from build123d import *

# Parameters (mm, degrees)
SKETCH1_W           = 2
SKETCH1_H           = 12
SKETCH1_W_2         = 19.5
SKETCH1_H_2         = 27
BOSS_EXTRUDE1_DEPTH = 4
SKETCH2_W           = 19.5
SKETCH2_H           = 5
SKETCH2_R           = 6
BOSS_EXTRUDE2_DEPTH = 16
BOSS_EXTRUDE3_START = 4
SKETCH3_R           = 10
BOSS_EXTRUDE3_DEPTH = 8
CHAMFER1_SIZE       = 1


with BuildPart() as part:
    # Sketch1 → Boss-Extrude1 (new body)
    with BuildSketch(Plane(origin=(0, 0, 0), x_dir=(1, 0, 0), z_dir=(0, 1, 0))):
        with Locations((-10.75, 0)):
            Rectangle(SKETCH1_W, SKETCH1_H)
        Rectangle(SKETCH1_W_2, SKETCH1_H_2)
        with Locations((10.75, 0)):
            Rectangle(SKETCH1_W, SKETCH1_H)
    extrude(amount=BOSS_EXTRUDE1_DEPTH)

    # Sketch2 → Boss-Extrude2 (add)
    with BuildSketch(Plane(origin=(0, 4, 0), x_dir=(1, 0, 0), z_dir=(0, 1, 0))):
        with BuildLine():
            Line((-6.373397172, 3.5), (-4.873397172, 3.5))
            ThreePointArc((-4.873397172, 3.5), (0, 6), (4.873397172, 3.5))
            Line((4.873397172, 3.5), (6.373397172, 3.5))
            Line((6.373397172, 3.5), (9.75, 8.5))
            Line((9.75, 8.5), (-9.75, 8.5))
            Line((-9.75, 8.5), (-6.373397172, 3.5))
        make_face()
        with Locations((0, 11)):
            Rectangle(SKETCH2_W, SKETCH2_H)
        Circle(SKETCH2_R)
        with BuildLine():
            Line((-6.373397172, -3.5), (-9.75, -8.5))
            Line((-9.75, -8.5), (9.75, -8.5))
            Line((9.75, -8.5), (6.373397172, -3.5))
            Line((6.373397172, -3.5), (4.873397172, -3.5))
            ThreePointArc((4.873397172, -3.5), (0, -6), (-4.873397172, -3.5))
            Line((-4.873397172, -3.5), (-6.373397172, -3.5))
        make_face()
        with Locations((0, -11)):
            Rectangle(SKETCH2_W, SKETCH2_H)
    extrude(amount=BOSS_EXTRUDE2_DEPTH)

    # Sketch3 → Boss-Extrude3 (add)
    with BuildSketch(Plane(origin=(0, 4, 0), x_dir=(1, 0, 0), z_dir=(0, 1, 0)).offset(BOSS_EXTRUDE3_START)):
        Circle(SKETCH3_R)
    extrude(amount=BOSS_EXTRUDE3_DEPTH)

    # Chamfer1
    chamfer1_edges = [part.edges().sort_by_distance(p)[0] for p in [
        (-9.75, 10, -13.5),
        (9.75, 10, -13.5),
        (9.75, 10, 13.5),
        (-9.75, 10, 13.5),
    ]]
    chamfer(chamfer1_edges, length=CHAMFER1_SIZE)


solid = part.part
For this review, take the finished solid that the model builds, in its own axes (mm). A direction names the side the tool comes from. Round coordinates to 2 decimals unless told otherwise and drop trailing zeros. Loops run counter-clockwise (first coordinate to the right, second up) from the corner with the lowest first, then second, coordinate; pieces in that order, holes last. Notation, with made-up numbers: (80, 87) - (137, 87) arc R9 ccw to (137, 103) - close; hole circle Ø6 at (-36, 75). An arc over 180 degrees is marked (long way). Use one line per item in the form item = value.
Item 1: Consider section C-C on z = -1.75. Write out the cut boundary in (x, y).
Answers:
outline = (-11.75, 0) - (11.75, 0) - (11.75, 4) - (5.74, 4) - (5.74, 8) - (9.85, 8) - (9.85, 16) - (5.74, 16) - (5.74, 20) - (-5.74, 20) - (-5.74, 16) - (-9.85, 16) - (-9.85, 8) - (-5.74, 8) - (-5.74, 4) - (-11.75, 4) - close
Item 2: Consider section D-D on y = 11.25. Write out the cut boundary in (x, z).
Answers:
outline = (-9.75, -12.5) - (-8.75, -13.5) - (8.75, -13.5) - (9.75, -12.5) - (9.75, -8.5) - (8.03, -5.96) arc R10 ccw to (8.03, 5.96) - (9.75, 8.5) - (9.75, 12.5) - (8.75, 13.5) - (-8.75, 13.5) - (-9.75, 12.5) - (-9.75, 8.5) - (-8.03, 5.96) arc R10 ccw to (-8.03, -5.96) - (-9.75, -8.5) - close
Item 3: Tool access review of faces 5 (the flat face through (9.75, 8, -10)), 6 (the cylindrical face through (10, 12, 0)), 7 (the flat face through (9, 4, 0)), 8 (the flat face through (-11, 2, -6)): name each direction out of +Z, -Z, +X, -X, +Y, -Y from which nothing blocks a thin tool from reaching the whole face with its end or side.
Answers:
face_5 = -Z, +X, +Y, -Y
face_6 = +X, +Y
face_7 = +X
face_8 = -Z, -X, +Y, -Y
Item 4: For line 1 (Y direction, x = 7.25, z = 0.25); line 2 (Z direction, x = 5, y = 7.75); line 3 (Z direction, x = 6.25, y = 5.75), list the stretches that pass through material, from the lowest coordinate up.
Answers:
line_1 = 0 to 4, 8 to 16
line_2 = -13.5 to -3.5, -3.32 to 3.32, 3.5 to 13.5
line_3 = -13.5 to -3.5, 3.5 to 13.5
Item 5: Clearance check with flat-ended pins moving along their axes: P1, Ø1.5, axis at x = -6.5, z = 1.5, coming from the +Y side; P2, Ø3, axis at y = 7.5, z = -6, coming from the +X side; P3, Ø3, axis at y = 14, z = -9, coming from the +X side; P4, Ø2, axis at x = 8.5, z = -3, coming from the +Y side. State where each tip first meets the part, or that it passes through.
Answers:
P1 = 20
P2 = 9.07
P3 = 9.75
P4 = 16
Item 6: Consider section A-A on y = 17.5. Write out the cut boundary in (x, z).
Answers:
outline = (-9.75, -12.5) - (-8.75, -13.5) - (8.75, -13.5) - (9.75, -12.5) - (9.75, -8.5) - (6.37, -3.5) - (4.87, -3.5) arc R6 ccw to (4.87, 3.5) - (6.37, 3.5) - (9.75, 8.5) - (9.75, 12.5) - (8.75, 13.5) - (-8.75, 13.5) - (-9.75, 12.5) - (-9.75, 8.5) - (-6.37, 3.5) - (-4.87, 3.5) arc R6 ccw to (-4.87, -3.5) - (-6.37, -3.5) - (-9.75, -8.5) - close
Item 7: Mouldability with a two-part tool opening along Y and no side actions: class faces 1 (the flat face through (8, 16, 0)), 2 (the flat face through (-8.4, 11.9, 6.5)), 3 (the flat face through (9.24, 9.86, 13.01)), 4 (the flat face through (-8, 8, 0)) as +Y half, -Y half, draft (parallel to the pull), parting line (faces both ways), or undercut.
Answers:
face_1 = +Y half
face_2 = undercut
face_3 = draft
face_4 = undercut
Item 8: Consider section B-B on x = 5.5. Write out the cut boundary in (y, z), then the cut area to 3 significant figures.
Answers:
outline = (0, -13.5) - (20, -13.5) - (20, -3.5) - (16, -3.5) - (16, -2.4) - (20, -2.4) - (20, 2.4) - (16, 2.4) - (16, 3.5) - (20, 3.5) - (20, 13.5) - (0, 13.5) - close; hole (4, -3.5) - (8, -3.5) - (8, -2.4) - (4, -2.4) - close; hole (4, 2.4) - (8, 2.4) - (8, 3.5) - (4, 3.5) - close
area = 522 mm^2
